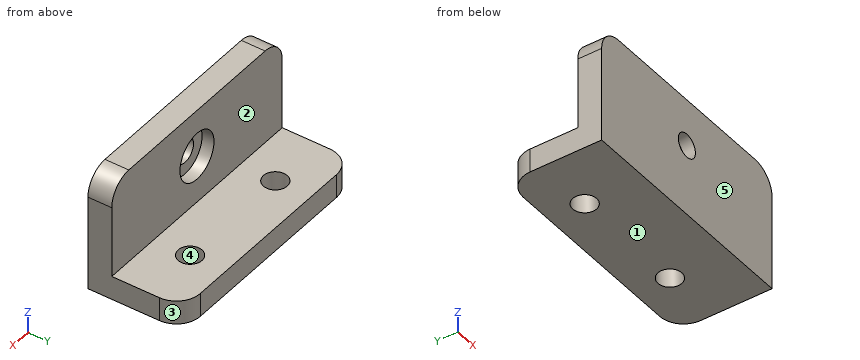
```python
from build123d import *

# Parameters (mm, degrees)
F0_W           = 100
F0_H           = 40
F1_DEPTH       = 5
F2_R           = 10
F3_W           = 100
F3_H           = 40
F4_DEPTH       = 10
F5_R           = 10
F8_D           = 10
F9_D           = 10
F9_CBORE_D     = 20
F9_CBORE_DEPTH = 5


with BuildPart() as f1:
    # F0 (on Front) → F1 (new body, symmetric)
    with BuildSketch(Plane.XZ):
        with Locations((0, 20)):
            Rectangle(F0_W, F0_H)
    extrude(amount=F1_DEPTH, both=True)

    # F2
    f2_edges = [f1.edges().sort_by_distance(p)[0] for p in [
        (-50, 0, 40),
        (50, 0, 40),
    ]]
    fillet(f2_edges, radius=F2_R)

    # F3 (on Top) → F4 (join)
    with BuildSketch(Plane.XY):
        with Locations((0, 15)):
            Rectangle(F3_W, F3_H)
    extrude(amount=-F4_DEPTH)

    # F5
    f5_edges = [f1.edges().sort_by_distance(p)[0] for p in [
        (-50, 35, -5),
        (50, 35, -5),
    ]]
    fillet(f5_edges, radius=F5_R)

    # F8 (through all)
    with Locations(Plane.XY):
        with Locations((25, 20), (-25, 20)):
            Hole(F8_D / 2)

    # F9 (through all)
    with Locations(Plane(origin=(0, 5, 0), x_dir=(-1, 0, 0), z_dir=(0, 1, 0))):
        with Locations((0, 20)):
            CounterBoreHole(F9_D / 2, F9_CBORE_D / 2, F9_CBORE_DEPTH)


solid = f1.part
```
Geometry check sheet. Reference: the model listing, model coordinates, mm. Face numbers are marked on the shaded views. A direction names the side the tool comes from. Coordinates: 2 decimals unless noted, no trailing zeros. Loops run counter-clockwise (first coordinate to the right, second up) from the corner with the lowest first, then second, coordinate; pieces in that order, holes last. Notation, with made-up numbers: (49, 32) - (82, 32) arc R11 ccw to (82, 41) - close; hole circle Ø5 at (31, 46.5). An arc over 180 degrees is marked (long way). One line per item, written item: value. Start each with the question number.
(1) Cross-section at C-C on z = -5.5. Enter the section's corners in (x, y).
(2) Cross-section at B-B on x = -25. Enter the section's corners in (y, z).
(3) Tool access check on the marked faces 1 and 2. Record the directions out of +Z, -Z, +X, -X, +Y, -Y that give a thin tool (end or side, any length) a straight path to the whole face; none if there is none.
(4) Depth check by flat-ended pin: P1, Ø1, axis at x = -12.5, y = 12, coming from the +Z side; P2, Ø20, axis at x = -0.5, z = 12, coming from the +Y side; P3, Ø10, axis at x = 1.5, z = 15.5, coming from the +Y side; P4, Ø6, axis at x = 0, z = 20, coming from the -Y side. Enter the tip coordinate at first touch or a pass-through.
(5) Material ranges on line 1 (Z direction, x = 0, y = 3.4); line 2 (Z direction, x = 0, y = -2.85); line 3 (Y direction, x = 25, z = -4.25), recorded low to high. Write a range as [from, to].
(6) Cross-section at A-A on y = 20. Enter the section's corners in (x, z).
(7) Cross-section at D-D on z = 23.5. Enter the section's corners in (x, y).
(8) Mould release check, pull along X, two halves, no side actions. Record for the marked faces 3, 4 and 5: released by +X, released by -X, zero draft, split by the parting line, or undercut.
Results below:
1. outline: (-50, -5) - (50, -5) - (50, 25) arc R10 ccw to (40, 35) - (-40, 35) arc R10 ccw to (-50, 25) - close; hole circle Ø10 at (-25, 20); hole circle Ø10 at (25, 20)
2. outline: (-5, -10) - (15, -10) - (15, 0) - (5, 0) - (5, 40) - (-5, 40) - close; (25, -10) - (35, -10) - (35, 0) - (25, 0) - close
3. face 1: -Z, +X, -X, +Y, -Y
3. face 2: +Z, +X, -X, +Y
4. P1: stops at z = 0
4. P2: stops at y = 5
4. P3: stops at y = 0
4. P4: passes through
5. line 1: z = [-10, 10], [30, 40]
5. line 2: z = [-10, 15], [25, 40]
5. line 3: y = [-5, 15], [25, 35]
6. outline: (-50, -10) - (-30, -10) - (-30, 0) - (-50, 0) - close; (-20, -10) - (20, -10) - (20, 0) - (-20, 0) - close; (30, -10) - (50, -10) - (50, 0) - (30, 0) - close
7. outline: (-50, -5) - (-3.57, -5) - (-3.57, 0) - (-9.37, 0) - (-9.37, 5) - (-50, 5) - close; (3.57, -5) - (50, -5) - (50, 5) - (9.37, 5) - (9.37, 0) - (3.57, 0) - close
8. face 3: released by +X
8. face 4: undercut
8. face 5: zero draft
